Autodesk Inventor part; units mm, degrees
ref_plane "YZ Plane" through (0, 0, 0) normal (1, 0, 0) x (0, 1, 0)
ref_plane "XZ Plane" through (0, 0, 0) normal (0, 1, 0) x (-1, 0, 0)
ref_plane "XY Plane" through (0, 0, 0) normal (0, 0, 1) x (1, 0, 0)
sketch "草图1" plane through (0, 0, 0) normal (0, 0, 1) x (1, 0, 0)
  circle A0 centre (0, 0) radius 1.05
  line L0 (1.1547, -2) -> (-1.1547, -2)
  line L1 (-1.1547, -2) -> (-2.3094, 0)
  line L2 (-2.3094, 0) -> (-1.1547, 2)
  line L3 (-1.1547, 2) -> (1.1547, 2)
  line L4 (1.1547, 2) -> (2.3094, 0)
  line L5 (2.3094, 0) -> (1.1547, -2)
  dimension "d0" = 2.1
  dimension "d2" = 4
extrude "拉伸1" add sketch "草图1" along normal blind 8 contours A0
extrude "拉伸2" add sketch "草图1" along normal blind 5
properties part number "铜柱"
The listing builds one solid part. Answer for the finished solid, in the listing's coordinates (mm). A direction names the side the tool comes from. Coordinates: 2 decimals unless noted, no trailing zeros. Write each loop counter-clockwise with the first axis right and the second up, starting at its lowest first coordinate (ties: lowest second). Pieces come first, ordered by that corner, then holes. Notation, with made-up numbers: (19.5, 57.5) - (23.5, 57.5) arc R14 ccw to (23.5, 74.5) - close; hole circle Ø3 at (3, 22.5). An arc over 180 degrees is marked (long way). Return JSON: item names as keys, results as strings. Group by question number.
Q1. The part is cut by section C-C on y = 0.1. Write down the section's boundary in (x, z).
Q2. The part is cut by section B-B on z = 3.75. Write down the section's boundary in (x, y).
Q3. Which of the six approach directions +Z, -Z, +X, -X, +Y, -Y give full straight-line access (tool end or side, diameter ignored) to faces 1 (the flat face through (-1, 1, 5)), 2 (the flat face through (0, -2, 2))?
Q4. The part is cut by section A-A on x = 0. Write down the section's boundary in (y, z), and give its area (3 significant figures).
Q5. The part is cut by section D-D on z = 6.75. Write down the section's boundary in (x, y), and give its area (3 significant figures).
Q6. A flat-ended cylindrical pin translates along its axis: pin 1 Ø1.5 at (x, y) = (-0.5, -1) entering from +Z. Find the tip coordinate at first contact, or state that the pin passes through.
Q7. Find the intervals of material crossed by line 1 along Z through (x, y) = (1, -1.7); line 2 along X through (y, z) = (-0.8, 1); line 3 along X through (y, z) = (-0.65, 4.75), in increasing order. Write a range as [from, to].
Evaluation:
{
 "1": {"outline": "(-2.25, 0) - (2.25, 0) - (2.25, 5) - (1.05, 5) - (1.05, 8) - (-1.05, 8) - (-1.05, 5) - (-2.25, 5) - close"},
 "2": {"outline": "(-2.31, 0) - (-1.15, -2) - (1.15, -2) - (2.31, 0) - (1.15, 2) - (-1.15, 2) - close"},
 "3": {"face 1": "+Z", "face 2": "+Z, -Z, +X, -X, -Y"},
 "4": {"outline": "(-2, 0) - (2, 0) - (2, 5) - (1.05, 5) - (1.05, 8) - (-1.05, 8) - (-1.05, 5) - (-2, 5) - close", "area": "26.3 mm2"},
 "5": {"outline": "circle Ø2.1 at (0, 0)", "area": "3.46 mm2"},
 "6": {"pin 1": "stops at z = 8"},
 "7": {"line 1": "z = [0, 5]", "line 2": "x = [-1.85, 1.85]", "line 3": "x = [-1.93, 1.93]"}
}
